```python
from build123d import *

# Parameters (mm, degrees)
F0_R     = 12.7
F0_R_2   = 10
F1_DEPTH = 290
F2_DEPTH = 76.2
F3_R     = 10
F4_DEPTH = 76.2
F5_R     = 2.5
F5_R_2   = 2.5019
F6_DEPTH = 63.5


with BuildPart() as f1:
    # F0 (on Front) → F1 (new body)
    with BuildSketch(Plane.XZ):
        Circle(F0_R)
        Circle(F0_R_2, mode=Mode.SUBTRACT)
        Circle(F0_R_2)
    extrude(amount=-F1_DEPTH)

    # F0 (on Front) → F2 (join)
    with BuildSketch(Plane.XZ):
        Circle(F0_R_2)
    extrude(amount=F2_DEPTH)

    # F3 (on face) → F4 (join)
    with BuildSketch(Plane(origin=(0, 290, 0), x_dir=(-1, 0, 0), z_dir=(0, 1, 0))):
        Circle(F3_R)
    extrude(amount=F4_DEPTH)

    # F5 (on Right) → F6 (cut, symmetric)
    with BuildSketch(Plane.YZ):
        with Locations((-64.77, 0)):
            Circle(F5_R)
        with Locations((354.77, 0)):
            Circle(F5_R_2)
    extrude(amount=F6_DEPTH, both=True, mode=Mode.SUBTRACT)


solid = f1.part
```
Build history of the part. All positions in model axes, mm. A direction names the side the tool comes from. Coordinates: 2 decimals unless noted, no trailing zeros. Order: outer loops, then holes, each group sorted by start corner. A loop starts at its lowest first (then second) coordinate and runs counter-clockwise, first axis right, second up. Notation, with made-up numbers: (-10, 40.5) -> (-4, 40.5) arc R23 ccw to (-4, 52.5) -> close; hole circle Ø1 at (86, -12.5). An arc over 180 degrees is marked (long way). Answer in a Markdown table with one row per item. Add a question column.
Q1. Band-saw the part on B-B, the plane y = 82.5. List the corners of the cut face in (x, z), then the cut area to 3 significant figures.
Q2. Band-saw the part on A-A, the plane x = -4.25. List the corners of the cut face in (y, z).
Q3. Wall check: line 1 along Y through (x, z) = (-1.5, 0.25); line 2 along Z through (x, y) = (8, -64.77); line 3 along Z through (x, y) = (-7, -64.77). Give the ranges that are in metal, low to high. Write a range as [from, to].
Q4. Drop flat-ended pins along their axis: pin 1 (6.5 mm diameter, centred on y = -64.77, z = 0, fed in from +X); pin 2 (6 mm diameter, centred on y = 103, z = -9.5, fed in from +X); pin 3 (3 mm diameter, centred on x = 3, y = 281.5, fed in from +Z). Give the stop position or say it passes through.
Q5. Which spindle directions (+Z, -Z, +X, -X, +Y, -Y) get a long thin tool onto all of the face, cutting with end or side? Do faces 1 (the face through (9.54, -37.57, 3)), 2 (the face through (-2.75, 142.97, -12.4)), 3 (the face through (-0.1, 290, -10.3)). Say none if no direction does.
Answers follow:
| question | item | result |
|---|---|---|
| 1 | outline | circle Ø25.4 at (0, 0) |
| 1 | area | 507 mm^2 |
| 2 | outline | (-76.2, -9.05) -> (0, -9.05) -> (0, -11.97) -> (290, -11.97) -> (290, -9.05) -> (366.2, -9.05) -> (366.2, 9.05) -> (290, 9.05) -> (290, 11.97) -> (0, 11.97) -> (0, 9.05) -> (-76.2, 9.05) -> close; hole circle Ø5 at (-64.77, 0); hole circle Ø5 at (354.77, 0) |
| 3 | line 1 | [-76.2, -67.26], [-62.28, 352.28], [357.26, 366.2] |
| 3 | line 2 | [-6, -2.5], [2.5, 6] |
| 3 | line 3 | [-7.14, -2.5], [2.5, 7.14] |
| 4 | pin 1 | x = 10 |
| 4 | pin 2 | x = 10.91 |
| 4 | pin 3 | z = 12.61 |
| 5 | face 1 | -Y |
| 5 | face 2 | +Y, -Y |
| 5 | face 3 | +Y |
